Geometry check sheet. Reference: drawing and pictorial views, mm from the part's lowest x, y, z. Give positions to 0.01 mm unless a question says otherwise; leave off trailing zeros. Write each loop counter-clockwise with the first axis right and the second up, starting at its lowest first coordinate (ties: lowest second). Pieces come first, ordered by that corner, then holes. Notation, with made-up numbers: (48.5, 36) -> (77.5, 36) arc R26 ccw to (77.5, 63) -> close; hole circle Ø10 at (27, 89.25). An arc over 180 degrees is marked (long way). Return JSON: item names as keys, results as strings.
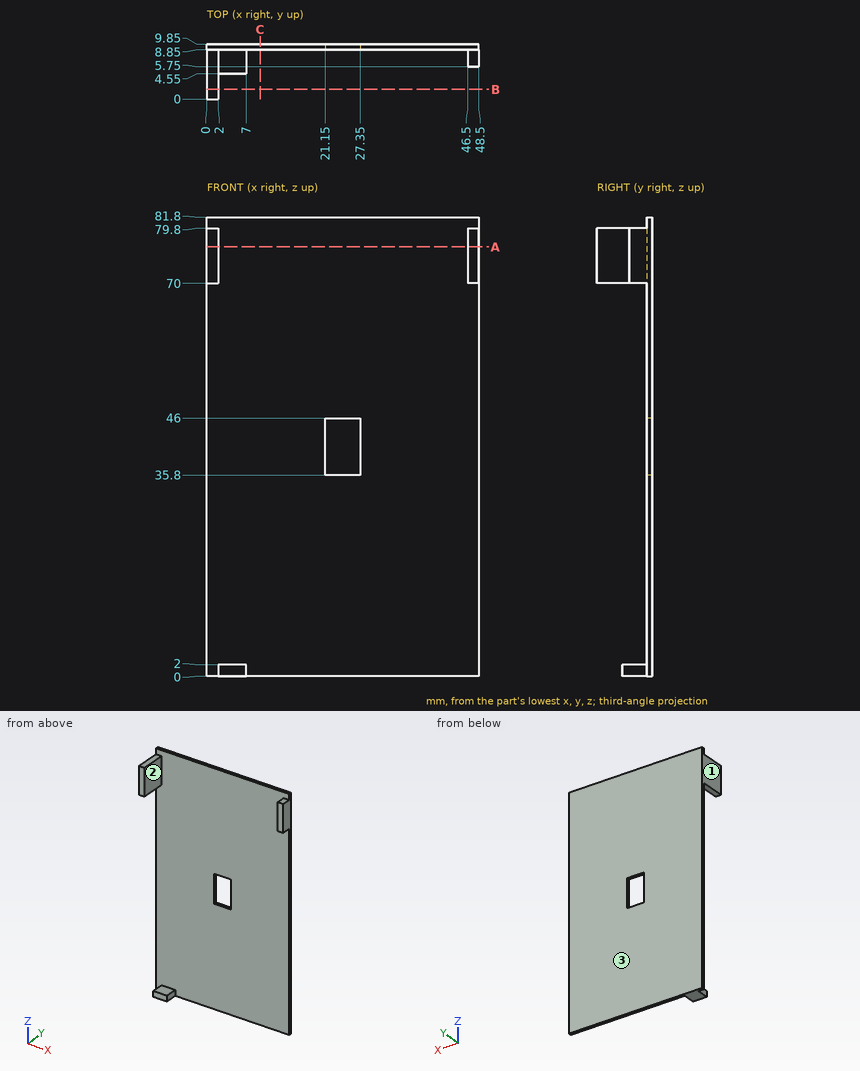
(1) Cross-section at A-A on z = 76.5. Enter the section's corners in (x, y), then the cut area to 3 significant figures.
Reply:
{"outline": "(0, 0) -> (2, 0) -> (2, 8.85) -> (46.5, 8.85) -> (46.5, 5.75) -> (48.5, 5.75) -> (48.5, 9.85) -> (0, 9.85) -> close", "area": "72.4 mm^2"}
(2) Depth check by flat-ended pin: pin 1 Ø0.6 at (y, z) = (6, 1) entering from +X; pin 2 Ø1.6 at (x, y) = (47.5, 7) entering from +Z; pin 3 Ø1 at (x, z) = (47.5, 73) entering from -Y; pin 4 Ø5 at (x, y) = (10.5, 2.5) entering from -Z. Enter the tip coordinate at first touch or a pass-through.
Reply:
{"pin 1": "x = 7", "pin 2": "z = 79.8", "pin 3": "y = 5.75", "pin 4": "through"}
(3) Thickness scan on L1, parallel to Y at x = 12.5, z = 39.5; L2, parallel to Z at x = 2.5, y = 8.5. Record the ranges inside material, lowest first.
Reply:
{"L1": "8.85 to 9.85", "L2": "0 to 2"}
(4) Release check for a two-part mould opening along X. For the marked faces 1, 2 and 3 record: pulls with the +X half, pulls with the -X half, needs draft (parallel to the pull), parting line crosses it, or undercut.
Reply:
{"face 1": "pulls with the -X half", "face 2": "undercut", "face 3": "needs draft"}
(5) Cross-section at B-B on y = 1.75. Enter the section's corners in (x, z), then the cut area to 3 significant figures.
Reply:
{"outline": "(0, 70) -> (2, 70) -> (2, 79.8) -> (0, 79.8) -> close", "area": "19.6 mm^2"}
(6) Cross-section at C-C on x = 9.5. Enter the section's corners in (y, z).
Reply:
{"outline": "(8.85, 0) -> (9.85, 0) -> (9.85, 81.8) -> (8.85, 81.8) -> close"}
